from build123d import *

# Parameters (mm, degrees)
SKETCH_R     = 40
PAD_DEPTH    = 37.4
POCKET_DEPTH = 37.401


with BuildPart() as part:
    # Sketch → Pad (new body)
    with BuildSketch(Plane.XY):
        with Locations((40, 0)):
            Circle(SKETCH_R)
    extrude(amount=PAD_DEPTH)

    # Sketch001 → Pocket (cut, through all)
    with BuildSketch(Plane.XY):
        Polygon((43.810512, 0), (41.905256, 3.3), (38.094744, 3.3), (36.189488, 0), (38.094744, -3.3), (41.905256, -3.3), align=None)
    extrude(amount=POCKET_DEPTH, mode=Mode.SUBTRACT)


solid = part.part
Can you work these out from the model? Positions are in its coordinate system, mm. A direction names the side the tool comes from. Round coordinates to 2 decimals unless told otherwise and drop trailing zeros. Loops run counter-clockwise (first coordinate to the right, second up) from the corner with the lowest first, then second, coordinate; pieces in that order, holes last. Notation, with made-up numbers: (66, -31.75) - (123, -31.75) arc R12 ccw to (123, -11.75) - close; hole circle Ø1 at (78.5, 17). An arc over 180 degrees is marked (long way). Answer in a Markdown table with one row per item. Add a question column.
Q1. I want a section at D-D on x = 13. List the corners of the cut face in (y, z) for me.
Q2. Which directions (+Z, -Z, +X, -X, +Y, -Y) give clear straight access to the entire face, cutting with the end or side of a thin tool? Please do faces 5 (the flat face through (42.87, 1.63, 18.44)), 6 (the flat face through (48, 1, 0)).
Q3. I want a section at B-B on z = 12. List the corners of the cut face in (x, y) for me.
Q4. I want a section at A-A on x = 40. List the corners of the cut face in (y, z) for me, and give its area (3 significant figures).
Q5. I need wall thicknesses on L1, parallel to Y at x = 41.5, z = 32; L2, parallel to Y at x = 42.5, z = 32; L3, parallel to Y at x = 19.5, z = 26.5. Which ranges of each line are inside material? Lowest first, please.
Q6. We'd pull the mould along X, two halves only. Please class faces 1 (the flat face through (40, 3.3, 18)), 2 (the flat face through (40, -3.3, 18)), 3 (the cylindrical face through (0.04, 1.76, 18.44)), 4 (the flat face through (48, 1, 37.4)): pulls with the +X half, pulls with the -X half, needs draft (parallel to the pull), parting line crosses it, or undercut.
Q7. I want a section at C-C on y = 11. List the corners of the cut face in (x, z) for me.
Q8. For pin 1 Ø4 at (y, z) = (-4.5, 8) entering from -X; pin 2 Ø6 at (x, z) = (43.5, 11) entering from -Y; pin 3 Ø1.5 at (y, z) = (-10, 10) entering from +X, each with a flat end and sliding along its axis, tell me the tip position at first contact or that it passes through.
A:
| question | item | result |
|---|---|---|
| 1 | outline | (-29.51, 0) - (29.51, 0) - (29.51, 37.4) - (-29.51, 37.4) - close |
| 2 | face 5 | +Z, -Z |
| 2 | face 6 | -Z, +X, -X, +Y, -Y |
| 3 | outline | circle Ø80 at (40, 0); hole (36.19, 0) - (38.09, -3.3) - (41.91, -3.3) - (43.81, 0) - (41.91, 3.3) - (38.09, 3.3) - close |
| 4 | outline | (-40, 0) - (-3.3, 0) - (-3.3, 37.4) - (-40, 37.4) - close; (3.3, 0) - (40, 0) - (40, 37.4) - (3.3, 37.4) - close |
| 4 | area | 2,750 mm^2 |
| 5 | L1 | -39.97 to -3.3, 3.3 to 39.97 |
| 5 | L2 | -39.92 to -2.27, 2.27 to 39.92 |
| 5 | L3 | -34.35 to 34.35 |
| 6 | face 1 | undercut |
| 6 | face 2 | undercut |
| 6 | face 3 | parting line crosses it |
| 6 | face 4 | needs draft |
| 7 | outline | (1.54, 0) - (78.46, 0) - (78.46, 37.4) - (1.54, 37.4) - close |
| 8 | pin 1 | x = 0.08 |
| 8 | pin 2 | y = -40 |
| 8 | pin 3 | x = 78.92 |
